Read the model definition and answer for the solid it produces. Units are mm, in the model's axes. Face numbers are marked on the shaded views. A direction names the side the tool comes from. Give positions to 0.01 mm unless a question says otherwise; leave off trailing zeros. Loops run counter-clockwise (first coordinate to the right, second up) from the corner with the lowest first, then second, coordinate; pieces in that order, holes last. Notation, with made-up numbers: (6.5, 44) - (33.5, 44) arc R14 cw to (33.5, 61) - close; hole circle Ø5 at (-24, 72.25). An arc over 180 degrees is marked (long way). Write item = value, one per line.
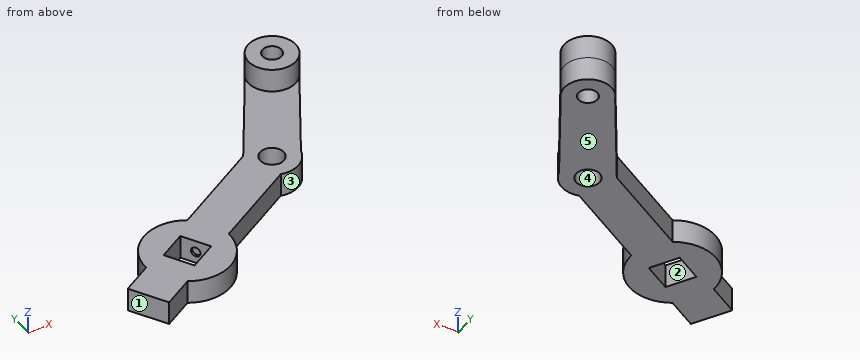
```python
from build123d import *

# Parameters (mm, degrees)
SKETCH1_R           = 2
SKETCH1_R_2         = 2.5
BOSS_EXTRUDE1_DEPTH = 5
SKETCH6_R           = 9
BOSS_EXTRUDE3_DEPTH = 5
CUT_EXTRUDE1_REACH  = 7
SKETCH13_R          = 1
CUT_EXTRUDE2_DEPTH  = 0.5
SKETCH14_R          = 5
SKETCH14_R_2        = 2
BOSS_EXTRUDE4_DEPTH = 5


with BuildPart() as part:
    # Sketch1 → Boss-Extrude1 (new body)
    with BuildSketch(Plane(origin=(0, 0, 0), x_dir=(0.498528904, -0.866873077, 0), z_dir=(0, 0, 1))):
        with BuildLine():
            Line((8.899126574, 3.869128256), (-2.35642803, 24.179978159))
            ThreePointArc((-2.35642803, 24.179978159), (-9.345167797, 25.255857552), (-10.421047189, 18.267117784))
            Line((-10.421047189, 18.267117784), (1.120951981, -3.909046337))
            ThreePointArc((1.120951981, -3.909046337), (8.899126574, -3.909046337), (8.899126574, 3.869128256))
        make_face()
        with Locations((-6.38873761, 21.223547972)):
            Circle(SKETCH1_R, mode=Mode.SUBTRACT)
        with Locations((5.010039278, -0.019959041)):
            Circle(SKETCH1_R_2, mode=Mode.SUBTRACT)
        with BuildLine():
            Line((8.899126574, -46.838046337), (8.899126574, -3.909046337))
            ThreePointArc((8.899126574, -3.909046337), (5.010039278, -5.519959041), (1.120951981, -3.909046337))
            Line((1.120951981, -3.909046337), (0.353553391, -2.434608777))
            Line((0.353553391, -2.434608777), (0.353553391, -46.838046337))
            Line((0.353553391, -46.838046337), (8.899126574, -46.838046337))
        make_face()
    extrude(amount=BOSS_EXTRUDE1_DEPTH)

    # Sketch6 → Boss-Extrude3 (add)
    with BuildSketch(Plane.XY.offset(5)):
        with Locations((-25.293181008, -19.882635909)):
            Circle(SKETCH6_R)
    extrude(amount=-BOSS_EXTRUDE3_DEPTH)

    # Sketch12 → Cut-Extrude1 (cut, up to next)
    with BuildSketch(Plane.XY.offset(5), mode=Mode.PRIVATE) as cut_extrude1_sk1:
        Polygon((-20.923894669, -21.061337265), (-24.114479652, -15.51334957), (-29.662467347, -18.703934553), (-26.471882365, -24.251922248), align=None)
    cut_extrude1_tool1 = extrude(cut_extrude1_sk1.sketch, amount=-CUT_EXTRUDE1_REACH, mode=Mode.PRIVATE) & part.part
    add(cut_extrude1_tool1.solids().sort_by_distance((-25.293181, -19.882636, 5))[0], mode=Mode.SUBTRACT)

    # Sketch13 → Cut-Extrude2 (cut)
    with BuildSketch(Plane(origin=(-24.825551359, -14.27689384, 0), x_dir=(0, 0, 1), z_dir=(-0.866873077, -0.498528904, 0))):
        with Locations((2.5, -4.626339983)):
            Circle(SKETCH13_R)
    extrude(amount=-CUT_EXTRUDE2_DEPTH, mode=Mode.SUBTRACT)

    # Sketch14 → Boss-Extrude4 (add)
    with BuildSketch(Plane.XY.offset(5)):
        with Locations((15.213151988, 16.118776732)):
            Circle(SKETCH14_R)
        with Locations((15.213151988, 16.118776732)):
            Circle(SKETCH14_R_2, mode=Mode.SUBTRACT)
    extrude(amount=BOSS_EXTRUDE4_DEPTH)


solid = part.part
```
1) Each of these flat-tipped pins is pushed along its axis until it touches: P1, Ø0.7, axis at x = 19.5, y = 13.5, coming from the -Z side; P2, Ø5, axis at y = 10, z = 1, coming from the -X side; P3, Ø6, axis at x = -4, z = 6, coming from the -Y side; P4, Ø5, axis at y = 2.5, z = 6, coming from the -X side. Where does it stop, or does it pass through?
Output:
P1 = 0
P2 = 3.83
P3 = -14.19
P4 = -0.83
2) The mould has two halves that part along Y. Classify the marked faces 3, 4 and 5: pulls with the +Y half, pulls with the -Y half, needs draft (parallel to the pull), parting line crosses it, or undercut.
Output:
face_3 = pulls with the -Y half
face_4 = undercut
face_5 = needs draft
3) A cutting plane is placed at A-A on x = 3. Determine the outline of the cut face in (y, z), then the cut area to 3 significant figures.
Output:
outline = (-9.83, 0) - (-6.8, 0) - (-6.8, 5) - (-9.83, 5) - close; (-1.91, 0) - (6.19, 0) - (6.19, 5) - (-1.91, 5) - close
area = 55.7 mm²
4) A cutting plane is placed at C-C on y = -25. Determine the outline of the cut face in (x, z), then the cut area to 3 significant figures.
Output:
outline = (-39.65, 0) - (-17.89, 0) - (-17.89, 5) - (-39.65, 5) - close
area = 109 mm²
5) A cutting plane is placed at D-D on x = -13.5. Determine the outline of the cut face in (y, z).
Output:
outline = (-18.03, 0) - (-8.17, 0) - (-8.17, 5) - (-18.03, 5) - close
6) A tool of negligible diameter and unlimited length cuts with its end or side. For the marked faces 1 and 2, from which of +Z, -Z, +X, -X, +Y, -Y can it reach the whole face along a straight path? Write none if from no direction.
Output:
face_1 = +Z, -Z, -X, -Y
face_2 = +Z, -Z
7) A cutting plane is placed at B-B on z = 7.5. Determine the outline of the cut face in (x, y).
Output:
outline = circle Ø10 at (15.21, 16.12); hole circle Ø4 at (15.21, 16.12)
8) Find the intervals of material crossed by probe 1 along Z at (x, y) = (-33.5, -22); probe 2 along X at (y, z) = (-3, 0.5); probe 3 along Y at (x, z) = (16.5, 3.75), in increasing order.
Output:
probe_1 = 0 to 5
probe_2 = -4.51 to 0.38, 4.58 to 9.47
probe_3 = 8.65 to 14.59, 17.65 to 20.95
